Read the model definition and answer for the solid it produces. Units are mm, in the model's axes. Face numbers are marked on the shaded views. A direction names the side the tool comes from. Coordinates: 2 decimals unless noted, no trailing zeros. Write each loop counter-clockwise with the first axis right and the second up, starting at its lowest first coordinate (ties: lowest second). Pieces come first, ordered by that corner, then holes.
1) Determine the mould class of the marked faces 5, 6 and 7 for opening direction Y: +Y half, -Y half, draft (parallel to the pull), parting line (faces both ways), or undercut.
2) Which of the six approach directions +Z, -Z, +X, -X, +Y, -Y give full straight-line access (tool end or side, diameter ignored) to the marked faces 1, 2, 3 and 4?
3) The part is cut by section B-B (y = -10). Determine the outline of the cut face in (x, z).
4) The part is cut by section C-C (z = -12). Determine the outline of the cut face in (x, y), then the cut area to 3 significant figures.
5) Each of these flat-tipped pins is pushed along its axis until it touches: pin 1 Ø1.6 at (x, z) = (-3, 1) entering from +Y; pin 2 Ø6 at (x, y) = (0, 27.5) entering from +Z; pin 3 Ø6 at (x, z) = (-25.5, -6) entering from +Y; pin 4 Ø3.5 at (y, z) = (24.5, -5.5) entering from -X. Where does it stop, or does it pass through?
6) The part is cut by section D-D (x = -8.5). Determine the outline of the cut face in (y, z), then the cut area to 3 significant figures.
7) The part is cut by section A-A (x = -23.2). Determine the outline of the cut face in (y, z).
8) Find the intervals of material crossed by line 1 (Y direction, x = 0, z = -11); line 2 (Y direction, x = -23.2, z = 0.05); line 3 (X direction, y = -8, z = -6.5), in increasing order.
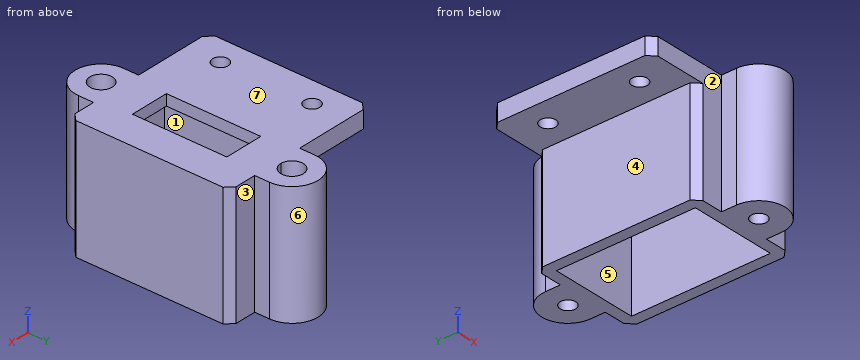
from build123d import *

# Parameters (mm, degrees)
F0_W     = 25
F0_H     = 40
F0_W_2   = 11.3
F0_H_2   = 27.175
F1_DEPTH = 3.2
F2_R     = 3.25
F2_W     = 25
F2_H     = 40
F3_DEPTH = 35
F4_W     = 15
F4_H     = 46.4
F4_R     = 2.25
F5_DEPTH = 5
F6_SIZE  = 2
F7_R     = 3.25
F7_R_2   = 2.25
F8_DEPTH = 3.2


with BuildPart() as f1:
    # F0 (on Top) → F1 (new body)
    with BuildSketch(Plane.XY):
        Rectangle(F0_W, F0_H)
        Rectangle(F0_W_2, F0_H_2, mode=Mode.SUBTRACT)
    extrude(amount=F1_DEPTH)

    # F2 (on face) → F3 (join)
    with BuildSketch(Plane.XY.offset(3.2)):
        with BuildLine():
            Line((15.7, -23.2), (15.7, 23.2))
            Line((15.7, 23.2), (7.5, 23.2))
            Line((7.5, 23.2), (7.5, 27.5))
            ThreePointArc((7.5, 27.5), (0, 35), (-7.5, 27.5))
            Line((-7.5, 27.5), (-7.5, 23.2))
            Line((-7.5, 23.2), (-15.7, 23.2))
            Line((-15.7, 23.2), (-15.7, -23.2))
            Line((-15.7, -23.2), (-7.5, -23.2))
            Line((-7.5, -23.2), (-7.5, -27.5))
            ThreePointArc((-7.5, -27.5), (0, -35), (7.5, -27.5))
            Line((7.5, -27.5), (7.5, -23.2))
            Line((7.5, -23.2), (15.7, -23.2))
        make_face()
        with Locations((0, -27.5)):
            Circle(F2_R, mode=Mode.SUBTRACT)
        Rectangle(F2_W, F2_H, mode=Mode.SUBTRACT)
        with BuildLine():
            ThreePointArc((0, 24.25), (-2.2980970389, 29.7980970389), (3.25, 27.5))
            ThreePointArc((3.25, 27.5), (2.2980970389, 25.2019029611), (0, 24.25))
        make_face(mode=Mode.SUBTRACT)
    extrude(amount=-F3_DEPTH)

    # F4 (on face) → F5 (join)
    with BuildSketch(Plane.XY.offset(3.2)):
        with Locations((-23.2, 0)):
            Rectangle(F4_W, F4_H)
        with Locations((-23.2, -13.2)):
            Circle(F4_R, mode=Mode.SUBTRACT)
        with Locations((-23.2, 13.2)):
            Circle(F4_R, mode=Mode.SUBTRACT)
    extrude(amount=-F5_DEPTH)

    # F6
    f6_edges = [f1.edges().sort_by_distance(p)[0] for p in [
        (15.7, 23.2, -14.3),
        (-15.7, 23.2, -16.8),
        (-15.7, -23.2, -16.8),
        (15.7, -23.2, -14.3),
        (-30.7, 23.2, 0.7),
        (-30.7, -23.2, 0.7),
    ]]
    chamfer(f6_edges, length=F6_SIZE)

    # F7 (on face) → F8 (join)
    with BuildSketch(Plane(origin=(0, 0, -31.8), x_dir=(1, 0, 0), z_dir=(0, 0, -1))):
        with Locations((0, -27.5)):
            Circle(F7_R)
        with Locations((0, -27.5)):
            Circle(F7_R_2, mode=Mode.SUBTRACT)
        with Locations((0, 27.5)):
            Circle(F7_R)
        with Locations((0, 27.5)):
            Circle(F7_R_2, mode=Mode.SUBTRACT)
    extrude(amount=-F8_DEPTH)


solid = f1.part
Reported:
1. face 5: undercut
1. face 6: +Y half
1. face 7: draft
2. face 1: -Z
2. face 2: +Z, -Z, -X, -Y
2. face 3: +Z, -Z, +X, +Y
2. face 4: -Z, -X, +Y, -Y
3. outline: (-30.7, -1.8) - (-15.7, -1.8) - (-15.7, -31.8) - (-12.5, -31.8) - (-12.5, 0) - (-5.65, 0) - (-5.65, 3.2) - (-30.7, 3.2) - close; (5.65, 0) - (12.5, 0) - (12.5, -31.8) - (15.7, -31.8) - (15.7, 3.2) - (5.65, 3.2) - close
4. outline: (-15.7, -21.2) - (-13.7, -23.2) - (-7.5, -23.2) - (-7.5, -27.5) arc R7.5 ccw to (7.5, -27.5) - (7.5, -23.2) - (13.7, -23.2) - (15.7, -21.2) - (15.7, 21.2) - (13.7, 23.2) - (7.5, 23.2) - (7.5, 27.5) arc R7.5 ccw to (-7.5, 27.5) - (-7.5, 23.2) - (-13.7, 23.2) - (-15.7, 21.2) - close; hole (-12.5, -20) - (12.5, -20) - (12.5, 20) - (-12.5, 20) - close; hole circle Ø6.5 at (0, -27.5); hole circle Ø6.5 at (0, 27.5)
4. area: 688 mm2
5. pin 1: stops at y = 34.67
5. pin 2: stops at z = -28.6
5. pin 3: passes through
5. pin 4: stops at x = -14.15
6. outline: (-23.2, -31.8) - (-20, -31.8) - (-20, 0) - (20, 0) - (20, -31.8) - (23.2, -31.8) - (23.2, 3.2) - (-23.2, 3.2) - close
6. area: 352 mm2
7. outline: (-23.2, -1.8) - (-15.45, -1.8) - (-15.45, 3.2) - (-23.2, 3.2) - close; (-10.95, -1.8) - (10.95, -1.8) - (10.95, 3.2) - (-10.95, 3.2) - close; (15.45, -1.8) - (23.2, -1.8) - (23.2, 3.2) - (15.45, 3.2) - close
8. line 1: y = -35 to -30.75, -24.25 to -20, 20 to 24.25, 30.75 to 35
8. line 2: y = -23.2 to -15.45, -10.95 to 10.95, 15.45 to 23.2
8. line 3: x = -15.7 to -12.5, 12.5 to 15.7
